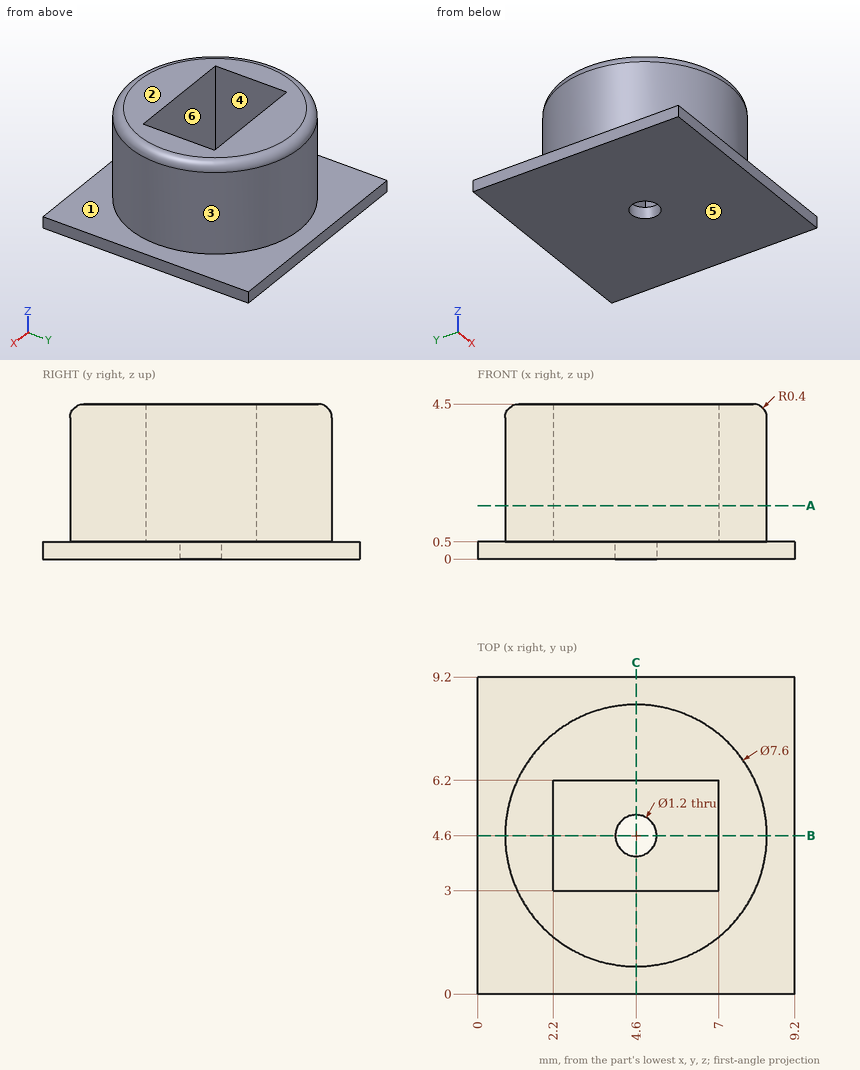
Can you work these out from the drawing? Everything is in mm from the part's minimum corner. A direction names the side the tool comes from. Round coordinates to 2 decimals unless told otherwise and drop trailing zeros. Order: outer loops, then holes, each group sorted by start corner. A loop starts at its lowest first (then second) coordinate and runs counter-clockwise, first axis right, second up. Notation, with made-up numbers: M 85.25,34 L 142.25,34 A21 ccw 142.25,55 Z; hole C 24.5,32.5 d11. An arc over 180 degrees is marked long. Answer as CSV lines item,"result".
Item 1: Imagine slicing it at A-A on z = 1.55. List the corners of the cut face in (x, y) for me.
From the geometry:
outline,"C 4.6,4.6 d7.6; hole M 2.2,3 L 7,3 L 7,6.2 L 2.2,6.2 Z"
Item 2: For pin 1 (1 mm diameter, centred on x = 1.5, z = 2, fed in from +Y); pin 2 (1.2 mm diameter, centred on x = 5, z = 3.5, fed in from +Y); pin 3 (1 mm diameter, centred on y = 5, z = 1.5, fed in from +X), each with a flat end and sliding along its axis, tell me the tip position at first contact or that it passes through.
From the geometry:
pin 1,"y = 7.37"
pin 2,"y = 8.4"
pin 3,"x = 8.4"
Item 3: Imagine slicing it at B-B on y = 4.6. List the corners of the cut face in (x, z) for me, and give its area (3 significant figures).
From the geometry:
outline,"M 0,0 L 4,0 L 4,0.5 L 2.2,0.5 L 2.2,4.5 L 1.2,4.5 A0.4 ccw 0.8,4.1 L 0.8,0.5 L 0,0.5 Z; M 5.2,0 L 9.2,0 L 9.2,0.5 L 8.4,0.5 L 8.4,4.1 A0.4 ccw 8,4.5 L 7,4.5 L 7,0.5 L 5.2,0.5 Z"
area,"15.1 mm2"
Item 4: Imagine slicing it at C-C on x = 4.6. List the corners of the cut face in (y, z) for me, and give its area (3 significant figures).
From the geometry:
outline,"M 0,0 L 4,0 L 4,0.5 L 3,0.5 L 3,4.5 L 1.2,4.5 A0.4 ccw 0.8,4.1 L 0.8,0.5 L 0,0.5 Z; M 5.2,0 L 9.2,0 L 9.2,0.5 L 8.4,0.5 L 8.4,4.1 A0.4 ccw 8,4.5 L 6.2,4.5 L 6.2,0.5 L 5.2,0.5 Z"
area,"21.5 mm2"
Item 5: Which directions (+Z, -Z, +X, -X, +Y, -Y) give clear straight access to the entire face, cutting with the end or side of a thin tool? Please do the marked faces 1 and 2.
From the geometry:
face 1,"+Z"
face 2,"+Z, +X, -X, +Y, -Y"
Item 6: Please list where these lines run through material, in increasing order: L1, parallel to Y at x = 4.5, z = 0.55; L2, parallel to Y at x = 4.6, z = 0.2; L3, parallel to X at y = 4.5, z = 2.75. Write a range as [from, to].
From the geometry:
L1,"[0.8, 3], [6.2, 8.4]"
L2,"[0, 4], [5.2, 9.2]"
L3,"[0.8, 2.2], [7, 8.4]"
Item 7: We'd pull the mould along X, two halves only. Please class the marked faces 3, 4, 5 and 6: +X half, -X half, draft (parallel to the pull), parting line (faces both ways), or undercut.
From the geometry:
face 3,"parting line"
face 4,"undercut"
face 5,"draft"
face 6,"undercut"
